The model under review builds one solid part; all positions refer to its coordinate system, in mm. Coordinates: 2 decimals unless noted, no trailing zeros. Order: outer loops, then holes, each group sorted by start corner. A loop starts at its lowest first (then second) coordinate and runs counter-clockwise, first axis right, second up. Notation, with made-up numbers: (-32.5, -10.5) -> (8.5, -10.5) arc R37 cw to (8.5, 25.5) -> close; hole circle Ø1 at (-6, -29.75). An arc over 180 degrees is marked (long way). Use CSV: the item, a comma, the result in double quotes. Start each with the question number.
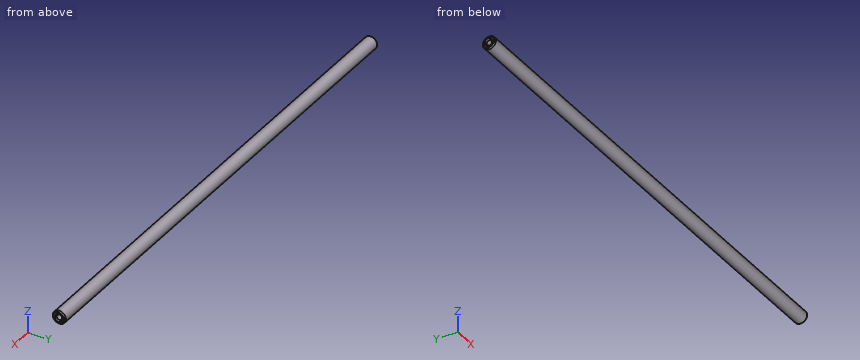
```python
from build123d import *

# Parameters (mm, degrees)
ESQUISSE1_R             = 4
BOSS_EXTRU_1_DEPTH      = 156
ESQUISSE2_R             = 1.65
ENL_V_MAT_EXTRU_1_DEPTH = 313
CHANFREIN1_SIZE         = 0.75


with BuildPart() as part:
    # Esquisse1 → Boss.-Extru.1 (new body, symmetric)
    with BuildSketch(Plane(origin=(0, 0, 0), x_dir=(0, 0, -1), z_dir=(1, 0, 0))):
        Circle(ESQUISSE1_R)
    extrude(amount=BOSS_EXTRU_1_DEPTH, both=True)

    # Esquisse2 → Enlèv. mat.-Extru.1 (cut, through all)
    with BuildSketch(Plane.ZY.offset(156)):
        Circle(ESQUISSE2_R)
    extrude(amount=-ENL_V_MAT_EXTRU_1_DEPTH, mode=Mode.SUBTRACT)

    # Chanfrein1
    chanfrein1_edges = [part.edges().sort_by_distance(p)[0] for p in [
        (-156, 0, 4),
        (156, 0, 4),
        (156, 0, -1.65),
        (-156, 0, -1.65),
    ]]
    chamfer(chanfrein1_edges, length=CHANFREIN1_SIZE)


solid = part.part
```
Q1. Add section A-A, the plane z = 0. State the section outline as (x, y) points.
Q2. To check wall thickness, follow probe 1 along Y at (x, z) = (10, 0); probe 2 along Y at (x, z) = (107.5, 1). State the ranges of each line that lie inside material, in increasing order.
Q3. Clearance check with flat-ended pins moving along their axes: pin 1 Ø1.5 at (x, z) = (122.5, 2) entering from -Y; pin 2 Ø4 at (y, z) = (0, 0) entering from +X. State where each tip first meets the part, or that it passes through.
Q4. Add section C-C, the plane x = 131.5. State the section outline as (y, z) points, then the cut area to 3 significant figures.
Answer block:
1,outline,"(-156, -3.25) -> (-155.25, -4) -> (155.25, -4) -> (156, -3.25) -> (156, -2.4) -> (155.25, -1.65) -> (-155.25, -1.65) -> (-156, -2.4) -> close; (-156, 2.4) -> (-155.25, 1.65) -> (155.25, 1.65) -> (156, 2.4) -> (156, 3.25) -> (155.25, 4) -> (-155.25, 4) -> (-156, 3.25) -> close"
2,probe 1,"y = -4 to -1.65, 1.65 to 4"
2,probe 2,"y = -3.87 to -1.31, 1.31 to 3.87"
3,pin 1,"stops at y = -3.8"
3,pin 2,"stops at x = 155.6"
4,outline,"circle Ø8 at (0, 0); hole circle Ø3.3 at (0, 0)"
4,area,"41.7 mm²"
